```python
from build123d import *

# Parameters (mm, degrees)
EXTRUDE_THIN1_DEPTH = 293.6875
FILLET1_R           = 1.27


with BuildPart() as part:
    # Sketch1 → Extrude-Thin1 (new body)
    with BuildSketch(Plane.XY):
        with BuildLine():
            Line((0, 0), (-6.35, 0))
            Line((-6.35, 0), (-6.35, 3.175))
            ThreePointArc((-6.35, 3.175), (-12.201824271, 10.612672966), (-14.2875, 19.84375))
            ThreePointArc((-14.2875, 19.84375), (-19.980512816, 23.16936432), (-22.225, 29.36875))
            Line((-22.225, 29.36875), (0, 29.36875))
            Line((0, 29.36875), (0, 28.09875))
            Line((0, 28.09875), (-20.85859868, 28.09875))
            ThreePointArc((-20.85859868, 28.09875), (-18.190231509, 23.133351298), (-12.986259744, 20.966776697))
            ThreePointArc((-12.986259744, 20.966776697), (-11.166701411, 11.396840635), (-5.08, 3.791149695))
            Line((-5.08, 3.791149695), (-5.08, 1.27))
            Line((-5.08, 1.27), (0, 1.27))
            Line((0, 1.27), (0, 0))
        make_face()
    extrude(amount=-EXTRUDE_THIN1_DEPTH)

    # Fillet1
    fillet1_edges = [part.edges().sort_by_distance(p)[0] for p in [
        (-12.986259744, 20.966776697, -146.84375),
        (-5.08, 3.791149695, -146.84375),
        (-6.35, 0, -146.84375),
        (-22.225, 29.36875, -146.84375),
    ]]
    fillet(fillet1_edges, radius=FILLET1_R)


solid = part.part
```
Geometry: final body of the model. Coordinates: model frame, mm. A direction names the side the tool comes from. Round coordinates to 2 decimals unless told otherwise and drop trailing zeros. Write each loop counter-clockwise with the first axis right and the second up, starting at its lowest first coordinate (ties: lowest second). Pieces come first, ordered by that corner, then holes.
Item 1: Set-up query: faces 4 (the face through (-3, 1.27, -145)), 5 (the face through (-19.431, 22.564, -144.788)). Return all of +Z, -Z, +X, -X, +Y, -Y with unobstructed straight access to the full face (end or side cutting, diameter ignored); none if empty.
Item 2: Section query A-A (x = -10). Return loops of the section in (y, z).
Item 3: Pin query (flat end, axial travel): P1, Ø1, axis at y = 2, z = -95.5, coming from the -X side; P2, Ø4, axis at x = -7.5, z = -185, coming from the -Y side; P3, Ø1.5, axis at x = -10, z = -243, coming from the -Y side; P4, Ø6, axis at x = -4, y = 7.5, coming from the +Z side. Return the tip coordinate at first contact, or that it passes through.
Item 4: Section query B-B (y = 6.75). Return loops of the section in (x, z), plus the area to 3 significant figures.
Item 5: Mould query, pull axis Y, two halves, no side actions, for faces 1 (the face through (-13.5, 18, -293.688)), 2 (the face through (-10, 28.099, -145)), 3 (the face through (-3, 0, -145)). Classes: +Y half, -Y half, draft (parallel to the pull), parting line (faces both ways), or undercut.
Item 6: Material intervals for L1, parallel to Y at x = -0.75, z = -55.5; L2, parallel to Y at x = -19.5, z = -85.5; L3, parallel to X at y = 2.75, z = -95, sorted ascending.
Completed:
1. face 4: +Z, -Z, +X
1. face 5: +Z, -Z, -X, -Y
2. outline: (6.97, -293.69) - (9.22, -293.69) - (9.22, 0) - (6.97, 0) - close; (28.1, -293.69) - (29.37, -293.69) - (29.37, 0) - (28.1, 0) - close
3. P1: stops at x = -6.35
3. P2: stops at y = 0.07
3. P3: stops at y = 6.03
3. P4: passes through
4. outline: (-9.83, -293.69) - (-8.2, -293.69) - (-8.2, 0) - (-9.83, 0) - close
4. area: 480 mm2
5. face 1: draft
5. face 2: undercut
5. face 3: -Y half
6. L1: y = 0 to 1.27, 28.1 to 29.37
6. L2: y = 22.63 to 24.64, 28.1 to 29.37
6. L3: x = -6.35 to -5.08
